The model under review builds one solid part; all positions refer to its coordinate system, in mm. A direction names the side the tool comes from. Give positions to 0.01 mm unless a question says otherwise; leave off trailing zeros. Write each loop counter-clockwise with the first axis right and the second up, starting at its lowest first coordinate (ties: lowest second). Pieces come first, ordered by that corner, then holes. Notation, with made-up numbers: (31, -1.75) - (70, -1.75) arc R32 cw to (70, 24.25) - close; hole circle Ø11 at (-29.5, 40). An arc over 180 degrees is marked (long way). Write item = value, one per line.
Autodesk Fusion 360 part; units mm, degrees
sketch "Sketch1" plane through (0, 0, 0) normal (0, 1, 0) x (1, 0, 0)
  line L0 (5, 0) -> (26.75, 0)
  line L1 (31.75, 5) -> (31.75, 76.2)
  line L2 (26.75, 76.2) -> (21.75, 76.2)
  line L3 (16.75, 71.2) -> (16.75, 71.2)
  line L4 (16.75, 71.2) -> (5, 71.2)
  line L5 (0, 66.2) -> (0, 66.2)
  line L6 (31.75, 71.2) -> (31.75, 66.2)
  line L7 (0, 66.2) -> (21.75, 66.2)
  line L8 (26.75, 61.2) -> (26.75, 36.75)
  line L9 (21.75, 31.75) -> (5, 31.75)
  line L10 (0, 26.75) -> (0, 5)
  arc A0 (21.75, 76.2) -> (16.75, 71.2) centre (21.75, 71.2) ccw
  arc A1 (31.75, 71.2) -> (26.75, 76.2) centre (26.75, 71.2) ccw
  arc A2 (5, 71.2) -> (0, 66.2) centre (5, 66.2) ccw
  arc A3 (26.75, 61.2) -> (21.75, 66.2) centre (21.75, 61.2) ccw
  arc A4 (21.75, 31.75) -> (26.75, 36.75) centre (21.75, 36.75) ccw
  arc A5 (5, 31.75) -> (0, 26.75) centre (5, 26.75) ccw
  arc A6 (0, 5) -> (5, 0) centre (5, 5) ccw
  arc A7 (26.75, 0) -> (31.75, 5) centre (26.75, 5) ccw
  circle A8 centre (15.875, 15.875) radius 12.5
  circle A9 centre (3.801, 3.801) radius 2.25
  dimension "d12" = 25
extrude "Extrude1" add sketch "Sketch1" along normal blind 5
sketch "Sketch2" plane through (0, 0, 0) normal (1, 0, 0) x (0, 0, -1)
1. Insertion check: P1, Ø2.5, axis at y = 2, z = -50.5, coming from the -X side; P2, Ø2.5, axis at x = 15, y = 2.5, coming from the -Z side; P3, Ø10, axis at x = 7, z = -33, coming from the -Y side. Each pin has a flat end and moves straight along its axis. Give the tip position at first contact, or say it passes through.
Findings below:
P1 = 26.75
P2 = -71.2
P3 = 0
2. Take a section at B-B on z = -9.5. Give the boundary of the cut face in (x, y), and give its area (3 significant figures).
Findings below:
outline = (0, 0) - (5.12, 0) - (5.12, 5) - (0, 5) - close; (26.63, 0) - (31.75, 0) - (31.75, 5) - (26.63, 5) - close
area = 51.2 mm²
3. Take a section at A-A on x = 20. Give the boundary of the cut face in (y, z).
Findings below:
outline = (0, -75.88) - (5, -75.88) - (5, -66.2) - (0, -66.2) - close; (0, -31.75) - (5, -31.75) - (5, -27.67) - (0, -27.67) - close; (0, -4.08) - (5, -4.08) - (5, 0) - (0, 0) - close
4. Machinability: for faces 1 (the flat face through (11, 2, -66.2)), 2 (the flat face through (18, 5, -30)), which of the approach directions +Z, -Z, +X, -X, +Y, -Y give a long, thin tool a straight path to every point of the face, cutting with its end or side? Answer none if there is none.
Findings below:
face_1 = -X, +Y, -Y
face_2 = +Z, -Z, +X, -X, +Y
5. Take a section at D-D on z = -23.5. Give the boundary of the cut face in (x, y), and give its area (3 significant figures).
Findings below:
outline = (0, 0) - (5.97, 0) - (5.97, 5) - (0, 5) - close; (25.78, 0) - (31.75, 0) - (31.75, 5) - (25.78, 5) - close
area = 59.7 mm²
6. For line 1 (Z direction, x = 16.5, y = 4.35); line 2 (Z direction, x = 23.5, y = 3); line 3 (X direction, y = 0.55, z = -5), list the stretches that pass through material, from the lowest coordinate up. Write a range as from..to.
Findings below:
line_1 = -71.2..-66.2, -31.75..-28.36, -3.39..0
line_2 = -76.2..-65.88, -32.07..-25.78, -5.97..0
line_3 = 0..1.9, 5.7..9.71, 22.04..31.75
7. Take a section at C-C on y = 1.2. Give the boundary of the cut face in (x, z) (3 decimals).
Findings below:
outline = (0, -66.2) arc R5 ccw to (5, -71.2) - (16.75, -71.2) arc R5 ccw to (21.75, -76.2) - (26.75, -76.2) arc R5 ccw to (31.75, -71.2) - (31.75, -5) arc R5 ccw to (26.75, 0) - (5, 0) arc R5 ccw to (0, -5) - (0, -26.75) arc R5 ccw to (5, -31.75) - (21.75, -31.75) arc R5 cw to (26.75, -36.75) - (26.75, -61.2) arc R5 cw to (21.75, -66.2) - close; hole circle Ø4.5 at (3.801, -3.801); hole circle Ø25 at (15.875, -15.875)
8. Draft analysis for pull direction Z (two halves, no side actions). For faces 3 (the flat face through (26.75, 2, -49)), 4 (the flat face through (11, 2, -71.2)), 5 (the cylindrical face through (25.32, 2.46, -33.25)), 6 (the flat face through (16, 2, 0)), state which applies: +Z half, -Z half, draft (parallel to the pull), parting line (faces both ways), or undercut.
Findings below:
face_3 = undercut
face_4 = -Z half
face_5 = undercut
face_6 = +Z half
